Autodesk Inventor part; units mm, degrees
ref_plane "YZ Plane" through (0, 0, 0) normal (1, 0, 0) x (0, 1, 0)
ref_plane "XZ Plane" through (0, 0, 0) normal (0, 1, 0) x (-1, 0, 0)
ref_plane "XY Plane" through (0, 0, 0) normal (0, 0, 1) x (1, 0, 0)
sketch "Sketch1" plane through (0, 0, 0) normal (0, 0, 1) x (1, 0, 0)
  line L0 (0, 0) -> (-100, 0)
  circle A0 centre (-100, -9) radius 1.5
  circle A1 centre (-16, -9) radius 1.5
  circle A2 centre (-58, -9) radius 1.5
  circle A3 centre (-58, -45) radius 1.5
  arc A4 (-100, 0) -> (-100, -18) centre (-100, -9) ccw
  arc A5 (-68, -45) -> (-48, -45) centre (-58, -45) ccw
  line L1 (0, -18) -> (-28, -18)
  line L2 (-28, -18) -> (-48, -38)
  line L3 (-48, -38) -> (-48, -45)
  line L4 (-68, -45) -> (-68, -18)
  line L5 (-68, -18) -> (-100, -18)
  line L6 (0, 0) -> (5, 0)
  line L7 (5, 0) -> (5, -18)
  line L8 (5, -18) -> (0, -18)
  dimension "d0" = 100
  dimension "d1" = 3
  dimension "d2" = 3
  dimension "d3" = 3
  dimension "d4" = 3
  dimension "d5" = 18
  dimension "d6" = 20
  dimension "d7" = 18
  dimension "d8" = 28
  dimension "d9" = 32
  dimension "d10" = 27
  dimension "d11" = 20
  dimension "d12" = 20
  dimension "d13" = 16
  dimension "d14" = 42
  dimension "d15" = 42
  dimension "d16" = 9
  dimension "d17" = 9
  dimension "d69" = 5
  dimension "d70" = 18
  dimension "d71" = 90
extrude "Extrusion7" add sketch "Sketch1" along normal blind 4
sketch "Sketch6" plane through (0, 0, 4) normal (0, 0, 1) x (1, 0, 0)
  line L0 (5, 0) -> (-100, 0)
  line L1 (5, 0) -> (-7, 0)
  line L2 (-7, 0) -> (-7, -18)
  line L3 (-7, -18) -> (5, -18)
  line L4 (5, -18) -> (5, 0)
  point P0 (0, 0)
  dimension "d74" = 12
  dimension "d75" = 18
extrude "Extrusion8" add sketch "Sketch6" along normal blind 14
shell "Shell6" thickness 4 removed faces 1 at (-3, -12, 18)
sketch "Sketch7" plane through (0, 0, 4) normal (0, 0, 1) x (1, 0, 0)
  point P0 (0, 0)
sketch "Sketch8" plane through (0, 0, 4) normal (0, 0, 1) x (1, 0, 0)
  point P0 (0, 0)
sketch "Sketch9" plane through (0, 0, 4) normal (0, 0, 1) x (1, 0, 0)
  circle A0 centre (-32, -9) radius 1.5
  circle A1 centre (-16, -9) radius 1.5
  line L0 (5, 0) -> (-7, 0)
  point P0 (0, 0)
  dimension "d79" = 3
  dimension "d80" = 16
  dimension "d81" = 9
extrude "Extrusion9" cut sketch "Sketch9" against normal through all contours A0
properties part number "Fall-Wk-3 - Mounting Bracket 1of3"
Check sheet for the modelled part. Datum: model origin and axes. Units: mm. A direction names the side the tool comes from. Round coordinates to 2 decimals unless told otherwise and drop trailing zeros. Loops run counter-clockwise (first coordinate to the right, second up) from the corner with the lowest first, then second, coordinate; pieces in that order, holes last. Notation, with made-up numbers: M 45.5,85 L 68.5,85 A33 ccw 68.5,114 Z; hole C -26,87 d9. An arc over 180 degrees is marked long. Answer as a JSON object with one key per item and string values.
1. Section check A-A (x = -32). Record the boundary of the cut face in (y, z), plus the area to 3 significant figures.
Reply:
{"outline": "M -22,0 L -10.5,0 L -10.5,4 L -22,4 Z; M -7.5,0 L 0,0 L 0,4 L -7.5,4 Z", "area": "76.0 mm²"}
2. Mould release check, pull along Y, two halves, no side actions. Record for faces 1 (the cylindrical face through (-56.614, -8.425, 1.972)), 2 (the flat face through (-4, -9, 18)), 3 (the cylindrical face through (-109, -9, 2)): pulls with the +Y half, pulls with the -Y half, needs draft (parallel to the pull), parting line crosses it, or undercut.
Reply:
{"face 1": "undercut", "face 2": "needs draft", "face 3": "parting line crosses it"}
3. Gauge pin test, flat ends, axial feed: P1, Ø3, axis at x = -65.5, y = -45.5, coming from the +Z side; P2, Ø3, axis at x = -97, z = 6.5, coming from the -Y side; P3, Ø1.2, axis at x = -84.5, z = 2, coming from the -Y side; P4, Ø4.5, axis at y = -27.5, z = 1, coming from the -X side. Record the tip position at first contact, or that the pin passes through.
Reply:
{"P1": "stops at z = 4", "P2": "passes through", "P3": "stops at y = -18", "P4": "stops at x = -68"}
4. Access from +Z, -Z, +X, -X, +Y, -Y to the whole of each face (thin tool, end or side, straight path). Record for faces 4 (the flat face through (-4, -18, 7)), 5 (the flat face through (-1, -9, 4)), 6 (the flat face through (-68, -32, 2)).
Reply:
{"face 4": "+Z, -Z, +X, -Y", "face 5": "+Z", "face 6": "+Z, -Z, -X, -Y"}
5. Scan lines: line 1 (Y direction, x = -58, z = 3.05); line 2 (X direction, y = -8, z = 5); line 3 (Y direction, x = -16, z = 1). Record each from-to range of solid material in increasing order.
Reply:
{"line 1": "y = -55 to -46.5, -43.5 to -10.5, -7.5 to 0", "line 2": "x = -7 to -3, 1 to 5", "line 3": "y = -18 to -10.5, -7.5 to 0"}
6. Section check D-D (z = 7.75). Record the boundary of the cut face in (x, y).
Reply:
{"outline": "M -7,-18 L 5,-18 L 5,0 L -7,0 Z; hole M -3,-14 L 1,-14 L 1,-4 L -3,-4 Z"}
7. Section check C-C (x = -58). Record the boundary of the cut face in (y, z), plus the area to 3 significant figures.
Reply:
{"outline": "M -55,0 L -46.5,0 L -46.5,4 L -55,4 Z; M -43.5,0 L -10.5,0 L -10.5,4 L -43.5,4 Z; M -7.5,0 L 0,0 L 0,4 L -7.5,4 Z", "area": "196 mm²"}
8. Section check B-B (y = -9). Record the boundary of the cut face in (x, z), plus the area to 3 significant figures.
Reply:
{"outline": "M -109,0 L -101.5,0 L -101.5,4 L -109,4 Z; M -98.5,0 L -59.5,0 L -59.5,4 L -98.5,4 Z; M -56.5,0 L -33.5,0 L -33.5,4 L -56.5,4 Z; M -30.5,0 L -17.5,0 L -17.5,4 L -30.5,4 Z; M -14.5,0 L 5,0 L 5,18 L 1,18 L 1,4 L -3,4 L -3,18 L -7,18 L -7,4 L -14.5,4 Z", "area": "520 mm²"}
